Build history of the part. All positions in model axes, mm. Face numbers are marked on the shaded views. A direction names the side the tool comes from. Coordinates: 2 decimals unless noted, no trailing zeros. Write each loop counter-clockwise with the first axis right and the second up, starting at its lowest first coordinate (ties: lowest second). Pieces come first, ordered by that corner, then holes.
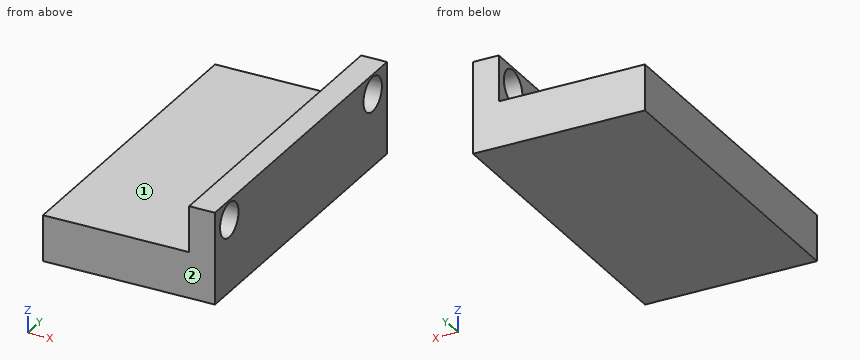
```python
from build123d import *

# Parameters (mm, degrees)
SKETCH2_W           = 10
SKETCH2_H           = 10
BOSS_EXTRUDE1_DEPTH = 5
SKETCH4_W           = 15
SKETCH4_H           = 27.94
BOSS_EXTRUDE4_DEPTH = 4
SKETCH5_W           = 2.25448465
SKETCH5_H           = 27.94
BOSS_EXTRUDE5_DEPTH = 4
SKETCH6_R           = 1.5
CUT_EXTRUDE1_DEPTH  = 40
SKETCH7_R           = 3.5
BOSS_EXTRUDE6_DEPTH = 8
SKETCH8_W           = 10
SKETCH8_H           = 10
CUT_EXTRUDE2_DEPTH  = 13


with BuildPart() as part:
    # Sketch2 → Boss-Extrude1 (new body)
    with BuildSketch(Plane.XY):
        with Locations((5, 5)):
            Rectangle(SKETCH2_W, SKETCH2_H)
    extrude(amount=BOSS_EXTRUDE1_DEPTH)

    # Sketch4 → Boss-Extrude4 (add)
    with BuildSketch(Plane.XY.offset(5)):
        with Locations((7.5, 5)):
            Rectangle(SKETCH4_W, SKETCH4_H)
    extrude(amount=BOSS_EXTRUDE4_DEPTH)

    # Sketch5 → Boss-Extrude5 (add)
    with BuildSketch(Plane.XY.offset(9)):
        with Locations((13.872757675, 5)):
            Rectangle(SKETCH5_W, SKETCH5_H)
    extrude(amount=BOSS_EXTRUDE5_DEPTH)

    # Sketch6 → Cut-Extrude1 (cut)
    with BuildSketch(Plane.ZY.offset(-12.74551535)):
        with Locations((11.286, 16.64426)):
            Circle(SKETCH6_R)
        with Locations((11.286, -6.645)):
            Circle(SKETCH6_R)
    extrude(amount=-CUT_EXTRUDE1_DEPTH, mode=Mode.SUBTRACT)

    # Sketch7 → Boss-Extrude6 (add)
    with BuildSketch(Plane(origin=(0, 0, 0), x_dir=(-1, 0, 0), z_dir=(0, 0, -1))):
        with Locations((-5, 5)):
            Circle(SKETCH7_R)
    extrude(amount=BOSS_EXTRUDE6_DEPTH)

    # Sketch8 → Cut-Extrude2 (cut)
    with BuildSketch(Plane(origin=(0, 0, -8), x_dir=(-1, 0, 0), z_dir=(0, 0, -1))):
        with Locations((-5, 5)):
            Rectangle(SKETCH8_W, SKETCH8_H)
    extrude(amount=-CUT_EXTRUDE2_DEPTH, mode=Mode.SUBTRACT)


solid = part.part
```
1. Saw through at B-B on y = -5.5. List the corners of the cut face in (x, z) (3 decimals), plus the area to 3 significant figures.
Computed values:
outline: (0, 5) - (15, 5) - (15, 10.317) - (12.746, 10.317) - (12.746, 9) - (0, 9) - close; (12.746, 12.255) - (15, 12.255) - (15, 13) - (12.746, 13) - close
area: 64.6 mm2
2. Probe line 1 along X through (y, z) = (-5.25, 12.5); line 2 along Z through (x, y) = (12, 2); line 3 along Y through (x, z) = (14.25, 11.5). List the from-to ranges inside material, lowest first.
Computed values:
line 1: x = 12.75 to 15
line 2: z = 5 to 9
line 3: y = -8.97 to -8.13, -5.16 to 15.16, 18.13 to 18.97
3. Saw through at A-A on z = 10.75. List the corners of the cut face in (x, y), plus the area to 3 significant figures.
Computed values:
outline: (12.75, -8.97) - (15, -8.97) - (15, -8.05) - (12.75, -8.05) - close; (12.75, -5.24) - (15, -5.24) - (15, 15.24) - (12.75, 15.24) - close; (12.75, 18.05) - (15, 18.05) - (15, 18.97) - (12.75, 18.97) - close
area: 50.4 mm2
4. Saw through at C-C on x = 14. List the corners of the cut face in (y, z) (3 decimals), plus the area to 3 significant figures.
Computed values:
outline: (-8.97, 5) - (18.97, 5) - (18.97, 13) - (-8.97, 13) - close; hole circle Ø3 at (-6.645, 11.286); hole circle Ø3 at (16.644, 11.286)
area: 209 mm2
5. 3-axis set-ups, long thin cutter, end or side, ignore diameter. For the marked faces 1 and 2: which of +Z, -Z, +X, -X, +Y, -Y reach the whole face in a straight line?
Computed values:
face 1: +Z, -X, +Y, -Y
face 2: +Z, -Z, +X, -X, -Y
6. Saw through at D-D on y = 5.5. List the corners of the cut face in (x, z).
Computed values:
outline: (0, 5) - (15, 5) - (15, 13) - (12.75, 13) - (12.75, 9) - (0, 9) - close
7. Flat gauge pins, fed straight in: pin 1 (1.5 mm diameter, centred on y = 8.5, z = 10.5, fed in from -X); pin 2 (3 mm diameter, centred on x = 11.5, z = 11.5, fed in from +Y); pin 3 (6 mm diameter, centred on x = 5, y = -4, fed in from +Z). Where does each tip first touch, or does it go through?
Computed values:
pin 1: stops at x = 12.75
pin 2: stops at y = 18.97
pin 3: stops at z = 9
